Job drawing, mm, ordinate dimensions from the low corner. One solid piece. A direction names the side the tool comes from. Coordinates: 2 decimals unless noted, no trailing zeros. Loops run counter-clockwise (first coordinate to the right, second up) from the corner with the lowest first, then second, coordinate; pieces in that order, holes last. Notation, with made-up numbers: M 88.5,17.5 L 138.5,17.5 A28 ccw 138.5,44.5 Z; hole C 4.5,22.5 d10. An arc over 180 degrees is marked long. Write each question's results on one line, items separated by ' | '. Start each with the question number.
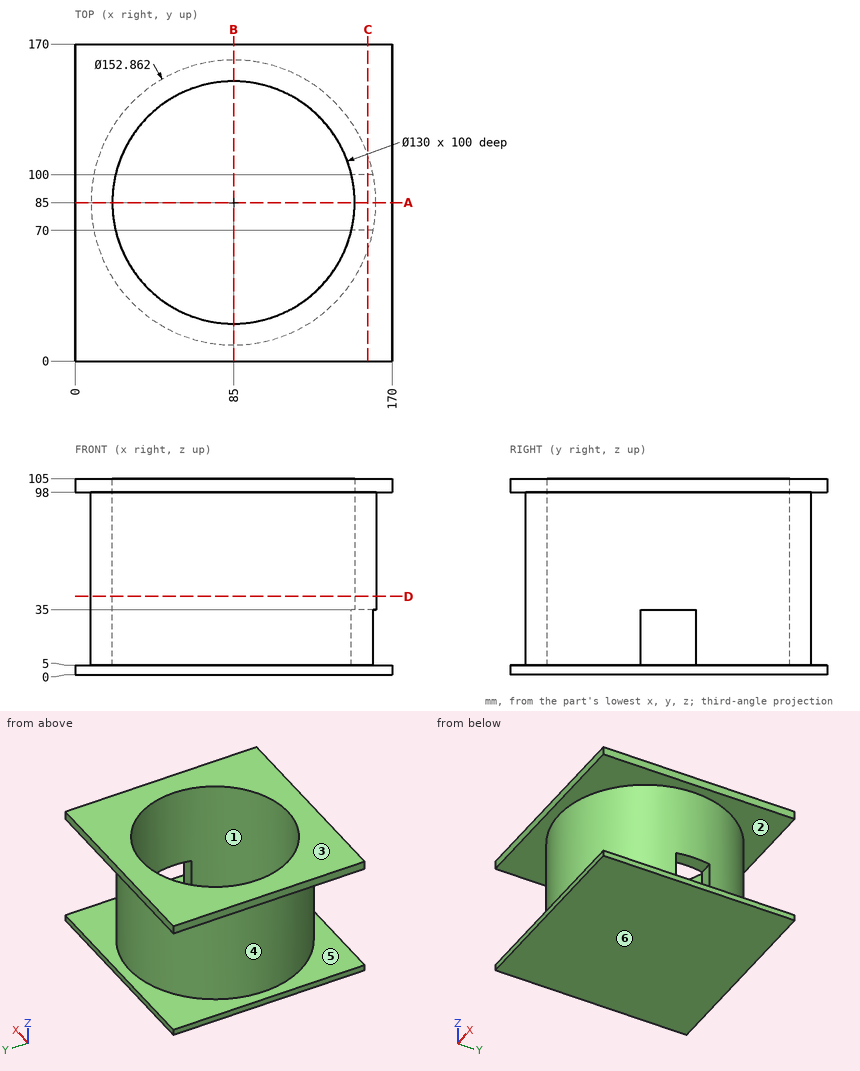
1. Band-saw the part on B-B, the plane x = 85. List the corners of the cut face in (y, z), plus the area to 3 significant figures.
2. Mould opens along Z. For the marked faces 3, 4, 5 and 6 say: +Z half, -Z half, draft (parallel to the pull), parting line (faces both ways), or undercut.
3. Band-saw the part on C-C, the plane x = 157. List the corners of the cut face in (y, z), plus the area to 3 significant figures.
4. Wall check: line 1 along Y through (x, z) = (85, 47); line 2 along Z through (x, y) = (47.5, 155); line 3 along Z through (x, y) = (75, 70). Give the ranges that are in metal, low to high.
5. Band-saw the part on D-D, the plane z = 42. List the corners of the cut face in (x, y), plus the area to 3 significant figures.
6. Which spindle directions (+Z, -Z, +X, -X, +Y, -Y) get a long thin tool onto all of the face, cutting with end or side? Do the marked faces 1 and 2. Say none if no direction does.
7. Pin check, flat tips, straight feed: pin 1 (1.5 mm diameter, centred on y = 125.5, z = 35.5, fed in from -X); pin 2 (13 mm diameter, centred on x = 157, z = 26, fed in from -Y); pin 3 (4 mm diameter, centred on y = 29.5, z = 63.5, fed in from -X) (1 decimal). Stop position of each tip, or through.
8. Band-saw the part on A-A, the plane y = 85. List the corners of the cut face in (x, z), plus the area to 3 significant figures.
Checked values:
1) outline: M 0,0 L 170,0 L 170,5 L 161.43,5 L 161.43,98 L 170,98 L 170,105 L 150,105 L 150,5 L 20,5 L 20,105 L 0,105 L 0,98 L 8.57,98 L 8.57,5 L 0,5 Z | area: 3,260 mm²
2) face 3: +Z half | face 4: undercut | face 5: undercut | face 6: -Z half
3) outline: M 0,0 L 170,0 L 170,5 L 110.65,5 L 110.65,98 L 170,98 L 170,105 L 0,105 L 0,98 L 59.35,98 L 59.35,5 L 0,5 Z; hole M 70,5 L 100,5 L 100,35 L 70,35 Z | area: 5,910 mm²
4) line 1: 8.57 to 20, 150 to 161.43 | line 2: 0 to 5, 98 to 105 | line 3: 0 to 5
5) outline: C 85,85 d152.86; hole C 85,85 d130 | area: 5,080 mm²
6) face 1: +Z | face 2: none
7) pin 1: x = 19.72 | pin 2: y = 45.61 | pin 3: x = 30.4
8) outline: M 0,0 L 170,0 L 170,5 L 20,5 L 20,105 L 0,105 L 0,98 L 8.57,98 L 8.57,5 L 0,5 Z; M 150,35 L 161.43,35 L 161.43,98 L 170,98 L 170,105 L 150,105 Z | area: 2,910 mm²
